from build123d import *

# Parameters (mm, degrees)
SKETCH1_R           = 25
BOSS_EXTRUDE1_DEPTH = 3
CUT_EXTRUDE1_DEPTH  = 3


with BuildPart() as part:
    # Sketch1 → Boss-Extrude1 (new body)
    with BuildSketch(Plane.XY):
        Circle(SKETCH1_R)
    extrude(amount=BOSS_EXTRUDE1_DEPTH)

    # Sketch2 → Cut-Extrude1 (cut)
    with BuildSketch(Plane(origin=(0, 0, 0), x_dir=(-1, 0, 0), z_dir=(0, 0, -1))):
        with BuildLine():
            Line((-24.979991994, -1), (-5, -1))
            Line((-5, -1), (-5, 1))
            Line((-5, 1), (-24.979991994, 1))
            ThreePointArc((-24.979991994, 1), (-25, 0), (-24.979991994, -1))
        make_face()
        with BuildLine():
            Line((5, 1), (5, -1))
            Line((5, -1), (24.979991994, -1))
            ThreePointArc((24.979991994, -1), (24.994997498, -0.50010007), (25, 0))
            ThreePointArc((25, 0), (24.994997498, 0.50010007), (24.979991994, 1))
            Line((24.979991994, 1), (5, 1))
        make_face()
    extrude(amount=-CUT_EXTRUDE1_DEPTH, mode=Mode.SUBTRACT)


solid = part.part
Work out the finished part from the listing and answer in its coordinate system (mm). A direction names the side the tool comes from. Coordinates: 2 decimals unless noted, no trailing zeros. Write each loop counter-clockwise with the first axis right and the second up, starting at its lowest first coordinate (ties: lowest second). Pieces come first, ordered by that corner, then holes.
1. For faces 4 (the flat face through (0, 0, 3)), 5 (the flat face through (5, 0, 1)), 6 (the flat face through (-5, 0, 1)), determine the directions among +Z, -Z, +X, -X, +Y, -Y from which every point of the face is accessible in a straight line to the end or side of a thin tool.
Results list:
face 4: +Z, +X, -X, +Y, -Y
face 5: +Z, -Z, +X
face 6: +Z, -Z, -X
2. Consider line 1 along Y through (x, z) = (8, 1.3); line 2 along Y through (x, z) = (22, 2.85); line 3 along X through (y, z) = (-18.5, 2.2). Determine where each line is inside the solid, lowest interval first.
Results list:
line 1: y = -23.69 to -1, 1 to 23.69
line 2: y = -11.87 to -1, 1 to 11.87
line 3: x = -16.82 to 16.82
3. The part is cut by section A-A, the plane z = 1.7. Write down the section's boundary in (x, y), and give its area (3 significant figures).
Results list:
outline: (-24.98, -1) arc R25 ccw to (24.98, -1) - (5, -1) - (5, 1) - (24.98, 1) arc R25 ccw to (-24.98, 1) - (-5, 1) - (-5, -1) - close
area: 1,880 mm2
4. The part is cut by section D-D, the plane x = 7.5. Write down the section's boundary in (y, z), and give its area (3 significant figures).
Results list:
outline: (-23.85, 0) - (-1, 0) - (-1, 3) - (-23.85, 3) - close; (1, 0) - (23.85, 0) - (23.85, 3) - (1, 3) - close
area: 137 mm2
5. The part is cut by section C-C, the plane y = 0. Write down the section's boundary in (x, z), and give its area (3 significant figures).
Results list:
outline: (-5, 0) - (5, 0) - (5, 3) - (-5, 3) - close
area: 30.0 mm2
6. For a pull along Y with two mould halves and no side action, classify faces 1 (the cylindrical face through (-0.536, -24.994, 1.479)), 2 (the flat face through (0, 0, 0)), 3 (the flat face through (-15, -1, 1)) as +Y half, -Y half, draft (parallel to the pull), parting line (faces both ways), or undercut.
Results list:
face 1: -Y half
face 2: draft
face 3: undercut
7. Flat-ended cylindrical pins translate along their axes: pin 1 (1.5 mm diameter, centred on x = 11.5, z = 2, fed in from +Y); pin 2 (0.9 mm diameter, centred on x = 13.5, z = 1, fed in from -Y); pin 3 (1.5 mm diameter, centred on x = -12, z = 2.5, fed in from +Y). Find the tip coordinate at first contact, or state that the pin passes through.
Results list:
pin 1: stops at y = 22.57
pin 2: stops at y = -21.32
pin 3: stops at y = 22.33
8. The part is cut by section B-B, the plane x = 16.5. Write down the section's boundary in (y, z).
Results list:
outline: (-18.78, 0) - (-1, 0) - (-1, 3) - (-18.78, 3) - close; (1, 0) - (18.78, 0) - (18.78, 3) - (1, 3) - close
